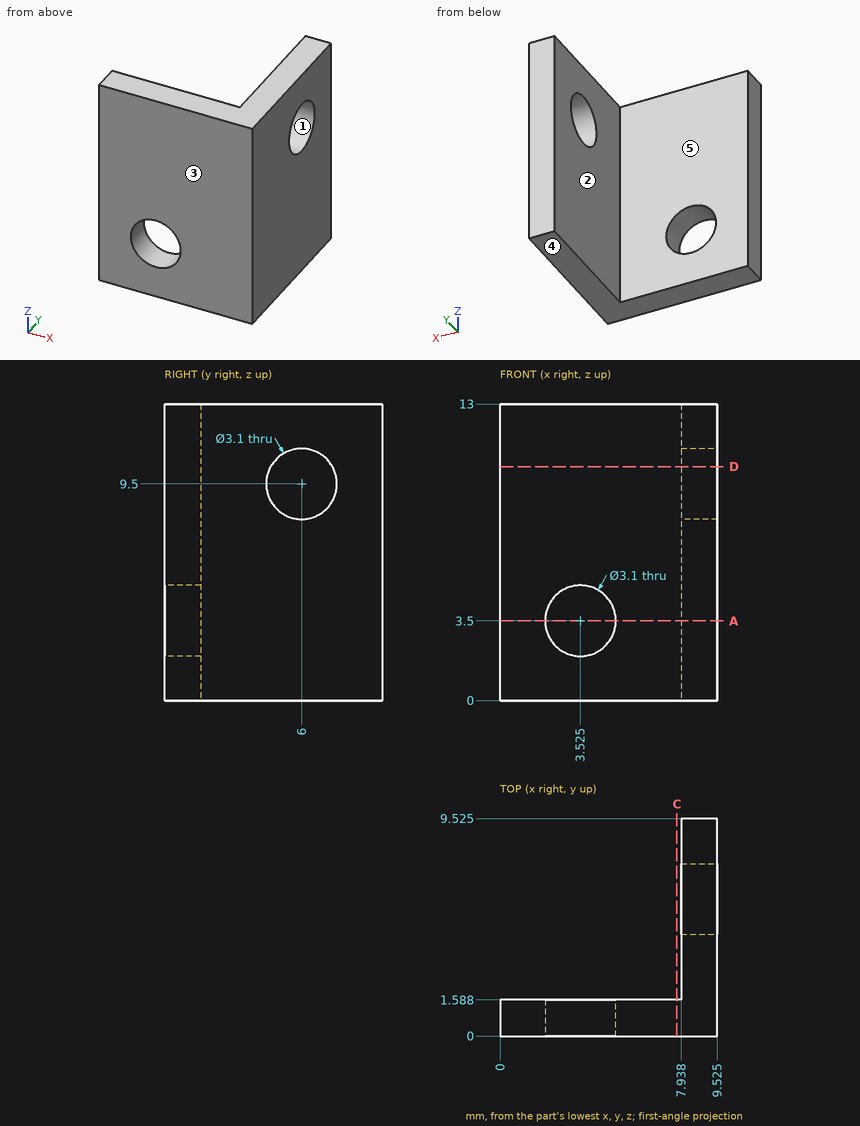
Here's the drawing with two shaded views (mm, measured from the low corner). I have some questions. A direction names the side the tool comes from. Coordinates: 2 decimals unless noted, no trailing zeros. Write each loop counter-clockwise with the first axis right and the second up, starting at its lowest first coordinate (ties: lowest second). Pieces come first, ordered by that corner, then holes. Notation, with made-up numbers: M 3.25,41 L 59.25,41 A26 cw 59.25,62 Z; hole C -2.5,-24.5 d9. An arc over 180 degrees is marked long. Use one line per item in the form item = value.
Q1. I need wall thicknesses on line 1 along Y through (x, z) = (7.5, 6.5); line 2 along X through (y, z) = (4.25, 8.5) (1 decimal); line 3 along Y through (x, z) = (8, 8.75) (1 decimal). Which ranges of each line are inside material? Lowest first, please. Write a range as from..to.
Model answer:
line_1 = 0..1.59
line_2 = 7.9..9.5
line_3 = 0..4.6, 7.4..9.5
Q2. We'd pull the mould along Y, two halves only. Please class the marked faces 1, 2 and 3: +Y half, -Y half, draft (parallel to the pull), parting line (faces both ways), or undercut.
Model answer:
face_1 = undercut
face_2 = draft
face_3 = -Y half
Q3. If we section it at A-A (z = 3.5): Write out the boundary of the cut face in (x, y) (1 decimal), then the cut area to 3 significant figures.
Model answer:
outline = M 0,0 L 2,0 L 2,1.6 L 0,1.6 Z; M 5.1,0 L 9.5,0 L 9.5,9.5 L 7.9,9.5 L 7.9,1.6 L 5.1,1.6 Z
area = 22.8 mm^2
Q4. For P1, Ø4, axis at y = 7, z = 9, coming from the -X side; P2, Ø4, axis at x = 2, y = 5, coming from the +Z side; P3, Ø1.5, axis at x = 1.5, z = 6.5, coming from the +Y side, each with a flat end and sliding along its axis, tell me the tip position at first contact or that it passes through.
Model answer:
P1 = 7.94
P2 = through
P3 = 1.59
Q5. For the marked faces 4 and 5, which set-ups out of +Z, -Z, +X, -X, +Y, -Y let a thin tool reach every point of the face, with its end or its side?
Model answer:
face_4 = -Z, +X, -X, +Y, -Y
face_5 = +Z, -Z, -X, +Y
Q6. If we section it at C-C (x = 7.75): Write out the boundary of the cut face in (y, z).
Model answer:
outline = M 0,0 L 1.59,0 L 1.59,13 L 0,13 Z
Q7. If we section it at D-D (z = 10.25): Write out the boundary of the cut face in (x, y) (1 decimal).
Model answer:
outline = M 0,0 L 9.5,0 L 9.5,4.6 L 7.9,4.6 L 7.9,1.6 L 0,1.6 Z; M 7.9,7.4 L 9.5,7.4 L 9.5,9.5 L 7.9,9.5 Z
